Here's how the part is built. I have some questions about the finished solid (model axes, mm). A direction names the side the tool comes from. Round coordinates to 2 decimals unless told otherwise and drop trailing zeros. Write each loop counter-clockwise with the first axis right and the second up, starting at its lowest first coordinate (ties: lowest second). Pieces come first, ordered by that corner, then holes. Notation, with made-up numbers: (62, -5) -> (69, -5) arc R23 ccw to (69, 30) -> close; hole circle Ø7 at (47.25, 64). An arc over 180 degrees is marked (long way). Put each result on its own line as item: value. Start each with the question number.
1. Which directions (+Z, -Z, +X, -X, +Y, -Y) give clear straight access to the entire face, cutting with the end or side of a thin tool? Please do faces 1 (the face through (15, -18, -39)), 2 (the face through (-10.88, 20.05, -17.59)), 3 (the face through (21.958, 6.345, -56.409)), 4 (the face through (-22.04, -1.95, -48.8)), 5 (the face through (0, 24, -7)).
2. Suppose I cut it at C-C (z = -45). Please give me the cut outline in (x, y).
3. I need wall thicknesses on probe 1 along Y at (x, z) = (16, -55); probe 2 along Z at (x, y) = (21.75, 0); probe 3 along X at (y, z) = (1, -39). Which ranges of each line are inside material? Lowest first, please. Write a range as from..to.
4. For pin 1 (7 mm diameter, centred on y = 0, z = -55, fed in from +X); pin 2 (4 mm diameter, centred on x = 14, z = -38.5, fed in from -Y); pin 3 (11 mm diameter, centred on x = 0, y = 0, fed in from -Z), each with a flat end and sliding along its axis, tell me the tip position at first contact or that it passes through.
5. Suppose I cut it at A-A (x = 0). Please give me the cut outline in (y, z).
6. We'd pull the mould along X, two halves only. Please class faces 6 (the face through (5.48, 3.11, -12.69)), 7 (the face through (-24.994, 0.536, -25.968)), 8 (the face through (14, 0, -46)), 9 (the face through (5, 0, 0)): +X half, -X half, draft (parallel to the pull), parting line (faces both ways), or undercut.
7. Suppose I cut it at B-B (z = -8.5). Please give me the cut outline in (x, y), then the cut area to 3 significant figures.
8. Suppose I cut it at D-D (x = 21.5). Please give me the cut outline in (y, z), then the cut area to 3 significant figures.
```python
from build123d import *

# Parameters (mm, degrees)
F0_R          = 25
F1_DEPTH      = 68
F3_DEPTH      = 25.001
F3_DEPTH_BACK = 25.001
F5_DEPTH      = 25.0010001
F5_DEPTH_BACK = 25.0010001
F8_R          = 4.25
F9_DEPTH      = 25
F12_DEPTH     = 10
F13_W         = 2
F13_H         = 2
F14_DEPTH     = 25


with BuildPart() as f1:
    # F0 (on Top) → F1 (new body)
    with BuildSketch(Plane.XY):
        Circle(F0_R)
    extrude(amount=-F1_DEPTH)

    # F2 (on Right) → F3 (cut, two sides)
    with BuildSketch(Plane.YZ) as f3_sk:
        with BuildLine():
            Line((-25, -15), (-28, -15))
            Line((-28, -15), (-28, -73))
            Line((-28, -73), (0, -73))
            Line((0, -73), (28, -73))
            Line((28, -73), (28, -15))
            Line((28, -15), (25, -15))
            ThreePointArc((25, -15), (20, -17.6457513111), (18, -22.9372539332))
            Line((18, -22.9372539332), (18, -55))
            ThreePointArc((18, -55), (14.1923881554, -64.1923881554), (5, -68))
            Line((5, -68), (0, -68))
            Line((0, -68), (-5, -68))
            ThreePointArc((-5, -68), (-14.1923881554, -64.1923881554), (-18, -55))
            Line((-18, -55), (-18, -22.9372539332))
            ThreePointArc((-18, -22.9372539332), (-20, -17.6457513111), (-25, -15))
        make_face()
    extrude(amount=-F3_DEPTH, mode=Mode.SUBTRACT)
    extrude(f3_sk.sketch, amount=F3_DEPTH_BACK, mode=Mode.SUBTRACT)

    # F4 (on Front) → F5 (cut, two sides)
    with BuildSketch(Plane.XZ) as f5_sk:
        with BuildLine():
            Line((14, -62.3349160121), (14, -29))
            ThreePointArc((14, -29), (0, -15), (-14, -29))
            Line((-14, -29), (-14, -62.3349160121))
            ThreePointArc((-14, -62.3349160121), (-14.0711119786, -62.9842348539), (-14.2810766389, -63.6027707973))
            Line((-14.2810766389, -63.6027707973), (-16.3315382908, -68))
            Line((-16.3315382908, -68), (16.3315382908, -68))
            Line((16.3315382908, -68), (14.2810766389, -63.6027707973))
            ThreePointArc((14.2810766389, -63.6027707973), (14.0711119786, -62.9842348539), (14, -62.3349160121))
        make_face()
    extrude(amount=-F5_DEPTH, mode=Mode.SUBTRACT)
    extrude(f5_sk.sketch, amount=F5_DEPTH_BACK, mode=Mode.SUBTRACT)

    # F6 (on Front) → F7 (revolve, cut)
    with BuildSketch(Plane.XZ):
        Polygon((-19, -48.5), (-26, -48.5), (-26, -55), (0, -55), (26, -55), (26, -48.5), (19, -48.5), (19, -51.8758), (0, -51.8758), (-19, -51.8758), align=None)
    revolve(axis=Axis((0.0713579357, 0, -55), (1, 0, 0)), mode=Mode.SUBTRACT)

    # F8 (on face) → F9 (cut)
    with BuildSketch(Plane.XY):
        Circle(F8_R)
    extrude(amount=-F9_DEPTH, mode=Mode.SUBTRACT)

    # F11 (on offset) → F12 (cut)
    with BuildSketch(Plane.XY.offset(-10)):
        Polygon((3.6373066959, -6.3), (7.2746133918, 0), (3.6373066959, 6.3), (-3.6373066959, 6.3), (-7.2746133918, 0), (-3.6373066959, -6.3), align=None)
    extrude(amount=-F12_DEPTH, mode=Mode.SUBTRACT)

    # F13 (on face) → F14 (cut)
    with BuildSketch(Plane.XY):
        with Locations((0, 25)):
            Rectangle(F13_W, F13_H)
        with Locations((0, -25)):
            Rectangle(F13_W, F13_H)
    extrude(amount=-F14_DEPTH, mode=Mode.SUBTRACT)


solid = f1.part
```
Verdict:
1. face 1: -Z, +X, -X, -Y
1. face 2: -Z, +X, -X, +Y
1. face 3: +X
1. face 4: -X
1. face 5: +Z, -Z, +Y
2. outline: (-17.35, -18) -> (-14, -18) -> (-14, 18) -> (-17.35, 18) arc R25 ccw to start; (14, -18) -> (17.35, -18) arc R25 ccw to (17.35, 18) -> (14, 18) -> close
3. probe 1: y = -18..-3.12, 3.12..18
3. probe 2: z = -68..-61.5, -48.5..0
3. probe 3: x = -24.98..-14, 14..24.98
4. pin 1: stops at x = 19
4. pin 2: stops at y = -18
4. pin 3: stops at z = -10
5. outline: (-24, -15) -> (-6.3, -15) -> (-6.3, -10) -> (-4.25, -10) -> (-4.25, 0) -> (-24, 0) -> close; (4.25, -10) -> (6.3, -10) -> (6.3, -15) -> (24, -15) -> (24, 0) -> (4.25, 0) -> close
6. face 6: undercut
6. face 7: -X half
6. face 8: undercut
6. face 9: draft
7. outline: (-1, -24.98) -> (-1, -24) -> (1, -24) -> (1, -24.98) arc R25 ccw to (1, 24.98) -> (1, 24) -> (-1, 24) -> (-1, 24.98) arc R25 ccw to start; hole circle Ø8.5 at (0, 0)
7. area: 1,900 mm^2
8. outline: (-12.76, -65.43) arc R13 ccw to (-5, -68) -> (5, -68) arc R13 ccw to (12.76, -65.43) -> (12.76, 0) -> (-12.76, 0) -> close; hole circle Ø13 at (0, -55)
8. area: 1,590 mm^2
